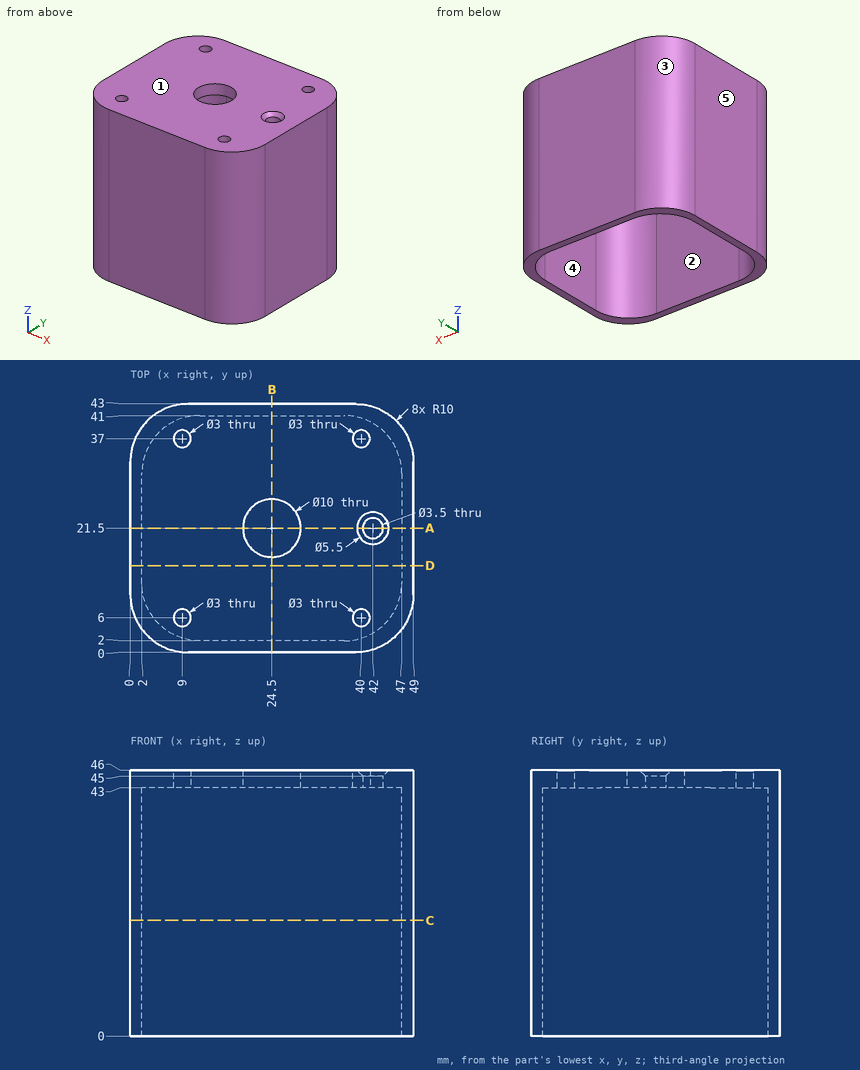
Design review of the part shown in the three views and the two pictorial views. Dimensions are in mm from the part's minimum x, y and z. A direction names the side the tool comes from. Round coordinates to 2 decimals unless told otherwise and drop trailing zeros. Order: outer loops, then holes, each group sorted by start corner. A loop starts at its lowest first (then second) coordinate and runs counter-clockwise, first axis right, second up. Notation, with made-up numbers: (82, 75.5) -> (126, 75.5) arc R29 ccw to (126, 101.5) -> close; hole circle Ø6 at (-16.5, -35.75). An arc over 180 degrees is marked (long way). Write item = value, one per line. Start each with the question number.
1) The part is to be moulded in two halves that separate along Y. For the marked faces 3, 4 and 5, say which applies: +Y half, -Y half, draft (parallel to the pull), parting line (faces both ways), or undercut.
2) Take a section at C-C on z = 20. State the section outline as (x, y) points.
3) Take a section at A-A on y = 21.5. State the section outline as (x, z) points.
4) Insertion check: pin 1 (3 mm diameter, centred on x = 23, y = 9, fed in from -Z); pin 2 (1.8 mm diameter, centred on x = 9, y = 6, fed in from +Z); pin 3 (4 mm diameter, centred on x = 44, z = 34.5, fed in from -Y). Each pin has a flat end and moves straight along its axis. Give the tip position at first contact, or say it passes through.
5) To check wall thickness, follow line 1 (X direction, y = 30.5, z = 40); line 2 (Y direction, x = 9, z = 44.95); line 3 (Y direction, x = 17, z = 41). State the ranges of each line that lie inside material, in increasing order. Write a range as from..to.
6) Take a section at D-D on y = 15. State the section outline as (x, z) points.
7) Tool access review of the marked faces 1 and 2: name each direction out of +Z, -Z, +X, -X, +Y, -Y from which nothing blocks a thin tool from reaching the whole face with its end or side.
8) Take a section at B-B on x = 24.5. State the section outline as (y, z) points, plus the area to 3 significant figures.
Verdict:
q1.face_3 = +Y half
q1.face_4 = undercut
q1.face_5 = draft
q2.outline = (0, 10) arc R10 ccw to (10, 0) -> (39, 0) arc R10 ccw to (49, 10) -> (49, 33) arc R10 ccw to (39, 43) -> (10, 43) arc R10 ccw to (0, 33) -> close; hole (2, 12) arc R10 ccw to (12, 2) -> (37, 2) arc R10 ccw to (47, 12) -> (47, 31) arc R10 ccw to (37, 41) -> (12, 41) arc R10 ccw to (2, 31) -> close
q3.outline = (0, 0) -> (2, 0) -> (2, 43) -> (19.5, 43) -> (19.5, 46) -> (0, 46) -> close; (29.5, 43) -> (40.25, 43) -> (40.25, 45) -> (39.25, 46) -> (29.5, 46) -> close; (43.75, 43) -> (47, 43) -> (47, 0) -> (49, 0) -> (49, 46) -> (44.75, 46) -> (43.75, 45) -> close
q4.pin_1 = 43
q4.pin_2 = through
q4.pin_3 = 0.46
q5.line_1 = 0..2, 47..49
q5.line_2 = 0.05..4.5, 7.5..35.5, 38.5..42.95
q5.line_3 = 0..2, 41..43
q6.outline = (0, 0) -> (2, 0) -> (2, 43) -> (47, 43) -> (47, 0) -> (49, 0) -> (49, 46) -> (0, 46) -> close
q7.face_1 = +Z, +X, -X, +Y, -Y
q7.face_2 = -Z
q8.outline = (0, 0) -> (2, 0) -> (2, 43) -> (16.5, 43) -> (16.5, 46) -> (0, 46) -> close; (26.5, 43) -> (41, 43) -> (41, 0) -> (43, 0) -> (43, 46) -> (26.5, 46) -> close
q8.area = 271 mm2
